from build123d import *

# Parameters (mm, degrees)
F0_W     = 113.393486
F0_H     = 135.465204
F1_DEPTH = 50
F2_W     = 95.314652
F2_H     = 121.38363
F3_DEPTH = 39.3
F5_DEPTH = 200


with BuildPart() as f1:
    # F0 (on Top) → F1 (new body)
    with BuildSketch(Plane.XY):
        Rectangle(F0_W, F0_H)
    extrude(amount=F1_DEPTH)

    # F2 (on face) → F3 (cut)
    with BuildSketch(Plane.XY.offset(50)):
        Rectangle(F2_W, F2_H)
    extrude(amount=-F3_DEPTH, mode=Mode.SUBTRACT)

    # F4 (on face) → F5 (cut)
    with BuildSketch(Plane(origin=(-56.696743, 0, 0), x_dir=(0, -1, 0), z_dir=(-1, 0, 0))):
        with BuildLine():
            ThreePointArc((-36.292743, 50), (-33.109312, 18.08902), (-5.88302, 35.035226))
            ThreePointArc((-5.88302, 35.035226), (-7.823794, 43.374538), (-13.247259, 50))
            Line((-13.247259, 50), (-36.292743, 50))
        make_face()
    extrude(amount=-F5_DEPTH, mode=Mode.SUBTRACT)


solid = f1.part
CAD build for the part. Positions are in the model's coordinates, mm. A direction names the side the tool comes from. Round coordinates to 2 decimals unless told otherwise and drop trailing zeros. Write each loop counter-clockwise with the first axis right and the second up, starting at its lowest first coordinate (ties: lowest second). Pieces come first, ordered by that corner, then holes.
(1) Slice it at A-A, the plane y = -41. Write the cut outline in (x, z), and give its area (3 significant figures).
(2) Slice it at D-D, the plane z = 44.5. Write the cut outline in (x, y).
(3) Slice it at C-C, the plane x = 22.5. Write the cut outline in (y, z).
(4) 3-axis set-ups, long thin cutter, end or side, ignore diameter. For faces 5 (the face through (-1, -67.733, 25)), 6 (the face through (47.657, -14, 31)): which of +Z, -Z, +X, -X, +Y, -Y reach the whole face in a straight line?
(5) Drop a flat-ended pin along its axis: P1, Ø5, axis at x = 6, y = -5.5, coming from the +Z side. Give the stop position or say it passes through.
(6) Slice it at B-B, the plane z = 19.5. Write the cut outline in (x, y).
(7) Mould opens along X. For faces 1 (the face through (-47.657, -14, 31)), 2 (the face through (0, -63, 50)), 3 (the face through (-1, 60.692, 31)), 4 (the face through (56.697, -1, 25)) say: pulls with the +X half, pulls with the -X half, needs draft (parallel to the pull), parting line crosses it, or undercut.
(8) Probe line 1 along Y through (x, z) = (-33, 45.5); line 2 along X through (y, z) = (-5, 21); line 3 along Z through (x, y) = (2.5, 2). List the from-to ranges inside material, lowest first.
From the geometry:
1. outline: (-56.7, 0) - (56.7, 0) - (56.7, 50) - (47.66, 50) - (47.66, 10.7) - (-47.66, 10.7) - (-47.66, 50) - (-56.7, 50) - close
1. area: 1,920 mm2
2. outline: (-56.7, -67.73) - (56.7, -67.73) - (56.7, 8.43) - (47.66, 8.43) - (47.66, -60.69) - (-47.66, -60.69) - (-47.66, 8.43) - (-56.7, 8.43) - close; (-56.7, 41.11) - (-47.66, 41.11) - (-47.66, 60.69) - (47.66, 60.69) - (47.66, 41.11) - (56.7, 41.11) - (56.7, 67.73) - (-56.7, 67.73) - close
3. outline: (-67.73, 0) - (67.73, 0) - (67.73, 50) - (60.69, 50) - (60.69, 10.7) - (-60.69, 10.7) - (-60.69, 50) - (-67.73, 50) - close
4. face 5: +Z, -Z, +X, -X, -Y
4. face 6: +Z
5. P1: stops at z = 10.7
6. outline: (-56.7, -67.73) - (56.7, -67.73) - (56.7, 14.03) - (47.66, 14.03) - (47.66, -60.69) - (-47.66, -60.69) - (-47.66, 14.03) - (-56.7, 14.03) - close; (-56.7, 35.51) - (-47.66, 35.51) - (-47.66, 60.69) - (47.66, 60.69) - (47.66, 35.51) - (56.7, 35.51) - (56.7, 67.73) - (-56.7, 67.73) - close
7. face 1: undercut
7. face 2: needs draft
7. face 3: undercut
7. face 4: pulls with the +X half
8. line 1: y = -67.73 to -60.69, 60.69 to 67.73
8. line 2: x = -56.7 to -47.66, 47.66 to 56.7
8. line 3: z = 0 to 10.7
